Read the model definition and answer for the solid it produces. Units are mm, in the model's axes. Give positions to 0.01 mm unless a question says otherwise; leave off trailing zeros. Order: outer loops, then holes, each group sorted by start corner. A loop starts at its lowest first (then second) coordinate and runs counter-clockwise, first axis right, second up. Notation, with made-up numbers: (19.5, 52) - (77.5, 52) arc R32 cw to (77.5, 87) - close; hole circle Ø5 at (75.25, 29.25). An arc over 180 degrees is marked (long way). Write each question's results on one line, items separated by ' | '.
Autodesk Inventor part; units mm, degrees
ref_plane "YZ Plane" through (0, 0, 0) normal (1, 0, 0) x (0, 1, 0)
ref_plane "XZ Plane" through (0, 0, 0) normal (0, 1, 0) x (-1, 0, 0)
ref_plane "XY Plane" through (0, 0, 0) normal (0, 0, 1) x (1, 0, 0)
sketch "Sketch1" plane through (0, 0, 0) normal (0, 0, 1) x (1, 0, 0)
  circle A0 centre (0, 0) radius 86
  circle A1 centre (0, 0) radius 140
  line L0 (98.9949, -98.9949) -> (-98.9949, 98.9949) construction
  line L1 (-98.9949, -98.9949) -> (98.9949, 98.9949) construction
  point P0 (0, 86)
  dimension "d44" = 172
  dimension "d23" = 280
extrude "Plate1" add sketch "Sketch1" along normal blind 4
sketch "Sketch6" plane through (0, 0, 0) normal (0, 0, 1) x (1, 0, 0)
  line L0 (0, 0) -> (0, 120) construction
  circle A0 centre (0, 0) radius 120 construction
  line L1 (0, 0) -> (84.8528, 84.8528) construction
  circle A1 centre (84.8528, 84.8528) radius 9
  dimension "d32" = 18
  dimension "d33" = 240
  dimension "d34" = 45
extrude "Cut2" cut sketch "Sketch6" along normal blind 4
pattern_circular "Circular Pattern2" count 8 over 360 about axis through (0, 0, -10) along (0, 0, -1) of "Cut2"
equation "\"d23\" = Flange_D_outer"
equation "\"d32\" = Flange_d_hole_diam"
equation "\"d33\" = Flange_D1_hole_center"
equation "\"d35\" = Thickness"
equation "\"d2\" = Thickness"
equation "\"BendReliefWidth\" = Thickness"
equation "\"BendReliefDepth\" = 0.5 * Thickness"
equation "\"CornerReliefSize\" = 4 * Thickness"
equation "\"MinimumRemnant\" = 2 * Thickness"
equation "\"TransitionRadius\" = BendRadius"
equation "\"JacobiRadiusSize\" = BendRadius"
equation "\"GapSize\" = Thickness"
equation "\"Octaeder_side\" = d41"
equation "\"Octaeder_flange_lenth\" = d42"
properties part number "DSB 112 drain system loose flange" material "Stainless Steel"
(1) Section C-C (x = -46) is taken. Give the vertices of the cut face in (y, z), plus the area to 3 significant figures.
Conclusion:
outline: (-132.23, 0) - (-72.66, 0) - (-72.66, 4) - (-132.23, 4) - close; (72.66, 0) - (132.23, 0) - (132.23, 4) - (72.66, 4) - close | area: 477 mm^2
(2) Section D-D (y = 53) is taken. Give the vertices of the cut face in (x, z), plus the area to 3 significant figures.
Conclusion:
outline: (-129.58, 0) - (-67.73, 0) - (-67.73, 4) - (-129.58, 4) - close; (67.73, 0) - (129.58, 0) - (129.58, 4) - (67.73, 4) - close | area: 495 mm^2
(3) Each of these flat-tipped pins is pushed along its axis until it touches: pin 1 (23.5 mm diameter, centred on x = -84.85, y = 84.85, fed in from +Z); pin 2 (2 mm diameter, centred on y = 31, z = 2.5, fed in from -X); pin 3 (14.5 mm diameter, centred on x = 120, y = 0, fed in from +Z); pin 4 (2 mm diameter, centred on x = 33.5, z = 1.5, fed in from +Y). Where does it stop, or does it pass through?
Conclusion:
pin 1: z = 4 | pin 2: x = -136.75 | pin 3: through | pin 4: y = 136.18
(4) Section A-A (y = 0) is taken. Give the vertices of the cut face in (x, z).
Conclusion:
outline: (-140, 0) - (-129, 0) - (-129, 4) - (-140, 4) - close; (-111, 0) - (-86, 0) - (-86, 4) - (-111, 4) - close; (86, 0) - (111, 0) - (111, 4) - (86, 4) - close; (129, 0) - (140, 0) - (140, 4) - (129, 4) - close
(5) Consider probe 1 along Y at (x, z) = (0, 1.65); probe 2 along X at (y, z) = (-90, 3.5); probe 3 along Y at (x, z) = (77, 2.75). Determine where each line is inside the solid, lowest interval first. Write a range as [from, to].
Conclusion:
probe 1: [-140, -129], [-111, -86], [86, 111], [129, 140] | probe 2: [-107.24, -92.24], [-77.47, 77.47], [92.24, 107.24] | probe 3: [-116.92, -89.25], [-80.46, -38.3], [38.3, 80.46], [89.25, 116.92]
(6) The mould has two halves that part along X. Classify faces 1 (the face through (113.362, 6.078, 1.972)), 2 (the face through (-111.1, 85.19, 1.97)), 3 (the face through (-64, -60, 0)): pulls with the +X half, pulls with the -X half, needs draft (parallel to the pull), parting line crosses it, or undercut.
Conclusion:
face 1: undercut | face 2: parting line crosses it | face 3: needs draft
